Here's how the part is built. I have some questions about the finished solid (model axes, mm). Face numbers are marked on the shaded views. A direction names the side the tool comes from. Give positions to 0.01 mm unless a question says otherwise; leave off trailing zeros. Loops run counter-clockwise (first coordinate to the right, second up) from the corner with the lowest first, then second, coordinate; pieces in that order, holes last. Notation, with made-up numbers: (18.25, 55) - (30.25, 55) arc R25 cw to (30.25, 72) - close; hole circle Ø3 at (-26.75, 50). An arc over 180 degrees is marked (long way). Return JSON: item names as keys, results as strings. Group by question number.
(1) If we section it at D-D (y = 17): Please give me the cut outline in (x, z).
(2) If we section it at B-B (y = 35): Please give me the cut outline in (x, z), then the cut area to 3 significant figures.
(3) I need wall thicknesses on probe 1 along X at (y, z) = (21.5, 7.5); probe 2 along Y at (x, z) = (8, 59); probe 3 along Y at (x, z) = (32.5, 44). Which ranges of each line are inside material? Lowest first, please. Write a range as [from, to].
(4) For P1, Ø12, axis at x = 24, y = 45, coming from the +Z side; P2, Ø5, axis at x = 27, y = 8.5, coming from the +Z side; P3, Ø9.5, axis at x = 29, y = 33.5, coming from the -Z side, each with a flat end and sliding along its axis, tell me the tip position at first contact or that it passes through.
(5) If we mould it in two halves opening along Z, with no side actions, what happens to the marked faces 1, 2 and 3? For each: released by +Z, released by -Z, zero draft, split by the parting line, or undercut.
(6) If we section it at A-A (x = 30): Please give me the cut outline in (y, z), then the cut area to 3 significant figures.
(7) On a 3-axis mill with a long thin cutter (end or side, diameter ignored), from which of +Z, -Z, +X, -X, +Y, -Y can I reach the whole of each face in a straight line? I mean the marked faces 4, 5 and 6. Say none if no direction works.
(8) If we section it at C-C (z = 21.5): Please give me the cut outline in (x, y), then the cut area to 3 significant figures.
```python
from build123d import *

# Parameters (mm, degrees)
SKIZZE1_W                          = 60
SKIZZE1_H                          = 70
GRUNDK_RPER_DEPTH                  = 60
FASE2_SIZE                         = 2
WANDUNG1_T                         = -4
SKIZZE2_W                          = 20
SKIZZE2_H                          = 6
AUFSATZ_LINEAR_AUSTRAGEN1_DEPTH    = 10
BOHRUNGEN_SERVO_REACH              = 106.929
SKIZZE3_R                          = 2.5
SECHSKANT_START                    = -4.2
SKIZZE5_R                          = 2.5
SKIZZE5_R_2                        = 2
SECHSKANT_DEPTH                    = 4.2
AUSPARUNGEN_DEPTH                  = 5
FASE3_SIZE                         = 7
BOHRUNGENHALTERUNG_REACH           = 112
SKIZZE8_R                          = 2
SECHSKANT_START_2                  = -9.5
SECHSKANT_DECKEL_DEPTH             = 9.5
BOHRUNG_VERSCHRAUBUNG_DECKEL_REACH = 112
SKIZZE11_R                         = 3
SKIZZE14_W                         = 12
SKIZZE14_H                         = 20
SKIZZE14_R                         = 0.883929471
VERTIEFUNG_DECKEL_DEPTH            = 2


with BuildPart() as part:
    # Skizze1 → Grundkörper (new body)
    with BuildSketch(Plane.XY):
        with Locations((30, 35)):
            Rectangle(SKIZZE1_W, SKIZZE1_H)
    extrude(amount=GRUNDK_RPER_DEPTH)

    # Fase2
    fase2_edges = [part.edges().sort_by_distance(p)[0] for p in [
        (30, 70, 0),
        (60, 35, 0),
        (0, 35, 0),
        (0, 70, 30),
        (60, 70, 30),
        (60, 0, 30),
        (0, 0, 30),
    ]]
    chamfer(fase2_edges, length=FASE2_SIZE)

    # Wandung1
    wandung1_openings = [part.faces().sort_by_distance(p)[0] for p in [
        (30, 35, 60),
    ]]
    offset(amount=WANDUNG1_T, openings=wandung1_openings)

    # Skizze2 → Aufsatz-Linear austragen1 (add)
    with BuildSketch(Plane(origin=(0, 4, 0), x_dir=(1, 0, 0), z_dir=(0, 1, 0))):
        with Locations((30, -47.1)):
            Rectangle(SKIZZE2_W, SKIZZE2_H)
    aufsatz_linear_austragen1 = extrude(amount=AUFSATZ_LINEAR_AUSTRAGEN1_DEPTH)

    # Spiegeln1: Aufsatz-Linear austragen1 across plane
    add(aufsatz_linear_austragen1.mirror(Plane(origin=(0, 35, 0), x_dir=(0, 0, 1), z_dir=(0, -1, 0))))

    # Skizze3 → Bohrungen Servo (cut, up to next)
    with BuildSketch(Plane.XY.offset(50.1), mode=Mode.PRIVATE) as bohrungen_servo_sk1:
        with Locations((25, 9)):
            Circle(SKIZZE3_R)
    bohrungen_servo_tool1 = extrude(bohrungen_servo_sk1.sketch, amount=-BOHRUNGEN_SERVO_REACH, mode=Mode.PRIVATE) & part.part
    # Skizze3 → Bohrungen Servo (cut, up to next)
    with BuildSketch(Plane.XY.offset(50.1), mode=Mode.PRIVATE) as bohrungen_servo_sk2:
        with Locations((35, 9)):
            Circle(SKIZZE3_R)
    bohrungen_servo_tool2 = extrude(bohrungen_servo_sk2.sketch, amount=-BOHRUNGEN_SERVO_REACH, mode=Mode.PRIVATE) & part.part
    # Skizze3 → Bohrungen Servo (cut, up to next)
    with BuildSketch(Plane.XY.offset(50.1), mode=Mode.PRIVATE) as bohrungen_servo_sk3:
        with Locations((35, 61)):
            Circle(SKIZZE3_R)
    bohrungen_servo_tool3 = extrude(bohrungen_servo_sk3.sketch, amount=-BOHRUNGEN_SERVO_REACH, mode=Mode.PRIVATE) & part.part
    # Skizze3 → Bohrungen Servo (cut, up to next)
    with BuildSketch(Plane.XY.offset(50.1), mode=Mode.PRIVATE) as bohrungen_servo_sk4:
        with Locations((25, 61)):
            Circle(SKIZZE3_R)
    bohrungen_servo_tool4 = extrude(bohrungen_servo_sk4.sketch, amount=-BOHRUNGEN_SERVO_REACH, mode=Mode.PRIVATE) & part.part
    add(bohrungen_servo_tool1.solids().sort_by_distance((25, 9, 50.1))[0], mode=Mode.SUBTRACT)
    add(bohrungen_servo_tool2.solids().sort_by_distance((35, 9, 50.1))[0], mode=Mode.SUBTRACT)
    add(bohrungen_servo_tool3.solids().sort_by_distance((35, 61, 50.1))[0], mode=Mode.SUBTRACT)
    add(bohrungen_servo_tool4.solids().sort_by_distance((25, 61, 50.1))[0], mode=Mode.SUBTRACT)

    # Skizze5 → Sechskant (cut)
    # profile 1 of 4: a face of its own
    with BuildSketch(Plane(origin=(0, 0, 44.1), x_dir=(-1, 0, 0), z_dir=(0, 0, -1)).offset(SECHSKANT_START)):
        Polygon((-34.978654144, 13.041395512), (-38.489278252, 11.03918381), (-38.510624109, 6.997788298), (-35.021345856, 4.958604488), (-31.510721748, 6.96081619), (-31.489375891, 11.002211702), align=None)
        with Locations(Location((-35, 9, 0), (0, 0, 180))):
            Circle(SKIZZE5_R, mode=Mode.SUBTRACT)
    # profile 2 of 4: a face of its own
    with BuildSketch(Plane(origin=(0, 0, 44.1), x_dir=(-1, 0, 0), z_dir=(0, 0, -1)).offset(SECHSKANT_START)):
        Polygon((-31.489375891, 58.997788298), (-34.978654144, 56.958604488), (-38.489278252, 58.96081619), (-38.510624109, 63.002211702), (-35.021345856, 65.041395512), (-31.510721748, 63.03918381), align=None)
        with Locations((-35, 61)):
            Circle(SKIZZE5_R, mode=Mode.SUBTRACT)
    # profile 3 of 4: a face of its own
    with BuildSketch(Plane(origin=(0, 0, 44.1), x_dir=(-1, 0, 0), z_dir=(0, 0, -1)).offset(SECHSKANT_START)):
        Polygon((-28.489278252, 63.03918381), (-28.510624109, 58.997788298), (-25.021345856, 56.958604488), (-21.510721748, 58.96081619), (-21.489375891, 63.002211702), (-24.978654144, 65.041395512), align=None)
        with Locations((-25, 61)):
            Circle(SKIZZE5_R, mode=Mode.SUBTRACT)
    # profile 4 of 4: a face of its own
    with BuildSketch(Plane(origin=(0, 0, 44.1), x_dir=(-1, 0, 0), z_dir=(0, 0, -1)).offset(SECHSKANT_START)):
        Polygon((-28.510624109, 11.002211702), (-25.021345856, 13.041395512), (-21.510721748, 11.03918381), (-21.489375891, 6.997788298), (-24.978654144, 4.958604488), (-28.489278252, 6.96081619), align=None)
        with Locations((-25, 9)):
            Circle(SKIZZE5_R_2, mode=Mode.SUBTRACT)
    extrude(amount=SECHSKANT_DEPTH, mode=Mode.SUBTRACT)

    # Skizze7 → Ausparungen (add)
    with BuildSketch(Plane.XY.offset(60)):
        Polygon((56, 4), (41, 4), (56, 19), align=None)
        Polygon((19, 4), (4, 19), (4, 4), align=None)
        Polygon((4, 66), (19, 66), (4, 51), align=None)
        Polygon((41, 66), (56, 51), (56, 66), align=None)
    extrude(amount=-AUSPARUNGEN_DEPTH)

    # Fase3
    fase3_edges = [part.edges().sort_by_distance(p)[0] for p in [
        (56, 11.5, 55),
        (48.5, 4, 55),
        (11.5, 4, 55),
        (4, 11.5, 55),
        (4, 58.5, 55),
        (11.5, 66, 55),
        (48.5, 66, 55),
        (56, 58.5, 55),
    ]]
    chamfer(fase3_edges, length=FASE3_SIZE)

    # Skizze8 → BohrungenHalterung (cut, up to next)
    with BuildSketch(Plane.XY.offset(60), mode=Mode.PRIVATE) as bohrungenhalterung_sk1:
        with Locations((52, 8)):
            Circle(SKIZZE8_R)
    bohrungenhalterung_tool1 = extrude(bohrungenhalterung_sk1.sketch, amount=-BOHRUNGENHALTERUNG_REACH, mode=Mode.PRIVATE) & part.part
    # Skizze8 → BohrungenHalterung (cut, up to next)
    with BuildSketch(Plane.XY.offset(60), mode=Mode.PRIVATE) as bohrungenhalterung_sk2:
        with Locations(Location((8, 8, 0), (0, 0, 45))):
            Circle(SKIZZE8_R)
    bohrungenhalterung_tool2 = extrude(bohrungenhalterung_sk2.sketch, amount=-BOHRUNGENHALTERUNG_REACH, mode=Mode.PRIVATE) & part.part
    # Skizze8 → BohrungenHalterung (cut, up to next)
    with BuildSketch(Plane.XY.offset(60), mode=Mode.PRIVATE) as bohrungenhalterung_sk3:
        with Locations((8, 62)):
            Circle(SKIZZE8_R)
    bohrungenhalterung_tool3 = extrude(bohrungenhalterung_sk3.sketch, amount=-BOHRUNGENHALTERUNG_REACH, mode=Mode.PRIVATE) & part.part
    # Skizze8 → BohrungenHalterung (cut, up to next)
    with BuildSketch(Plane.XY.offset(60), mode=Mode.PRIVATE) as bohrungenhalterung_sk4:
        with Locations(Location((52, 62, 0), (0, 0, 45))):
            Circle(SKIZZE8_R)
    bohrungenhalterung_tool4 = extrude(bohrungenhalterung_sk4.sketch, amount=-BOHRUNGENHALTERUNG_REACH, mode=Mode.PRIVATE) & part.part
    add(bohrungenhalterung_tool1.solids().sort_by_distance((52, 8, 60))[0], mode=Mode.SUBTRACT)
    add(bohrungenhalterung_tool2.solids().sort_by_distance((8, 8, 60))[0], mode=Mode.SUBTRACT)
    add(bohrungenhalterung_tool3.solids().sort_by_distance((8, 62, 60))[0], mode=Mode.SUBTRACT)
    add(bohrungenhalterung_tool4.solids().sort_by_distance((52, 62, 60))[0], mode=Mode.SUBTRACT)

    # Skizze13 → Sechskant Deckel (cut)
    with BuildSketch(Plane.XY.offset(57.5).offset(SECHSKANT_START_2)):
        Polygon((50.909166509, 57.928953988), (54.98021252, 59.01978748), (56.071046012, 63.090833491), (53.090833491, 66.071046012), (49.01978748, 64.98021252), (47.928953988, 60.909166509), align=None)
        Polygon((49.01978748, 5.01978748), (53.090833491, 3.928953988), (56.071046012, 6.909166509), (54.98021252, 10.98021252), (50.909166509, 12.071046012), (47.928953988, 9.090833491), align=None)
        Polygon((3.928953988, 6.909166509), (6.909166509, 3.928953988), (10.98021252, 5.01978748), (12.071046012, 9.090833491), (9.090833491, 12.071046012), (5.01978748, 10.98021252), align=None)
        Polygon((5.01978748, 59.01978748), (9.090833491, 57.928953988), (12.071046012, 60.909166509), (10.98021252, 64.98021252), (6.909166509, 66.071046012), (3.928953988, 63.090833491), align=None)
    extrude(amount=SECHSKANT_DECKEL_DEPTH, mode=Mode.SUBTRACT)

    # Skizze11 → Bohrung Verschraubung Deckel (cut, up to next)
    with BuildSketch(Plane(origin=(0, 0, 0), x_dir=(-1, 0, 0), z_dir=(0, 0, -1)), mode=Mode.PRIVATE) as bohrung_verschraubung_deckel_sk1:
        with Locations((-30, 35)):
            Circle(SKIZZE11_R)
    bohrung_verschraubung_deckel_tool1 = extrude(bohrung_verschraubung_deckel_sk1.sketch, amount=-BOHRUNG_VERSCHRAUBUNG_DECKEL_REACH, mode=Mode.PRIVATE) & part.part
    add(bohrung_verschraubung_deckel_tool1.solids().sort_by_distance((30, 35, 0))[0], mode=Mode.SUBTRACT)

    # Skizze14 → Vertiefung Deckel (cut)
    with BuildSketch(Plane(origin=(0, 0, 0), x_dir=(-1, 0, 0), z_dir=(0, 0, -1))):
        with Locations((-30, 30)):
            Rectangle(SKIZZE14_W, SKIZZE14_H)
        with Locations((-30, 35)):
            Circle(SKIZZE14_R, mode=Mode.SUBTRACT)
    extrude(amount=-VERTIEFUNG_DECKEL_DEPTH, mode=Mode.SUBTRACT)


solid = part.part
```
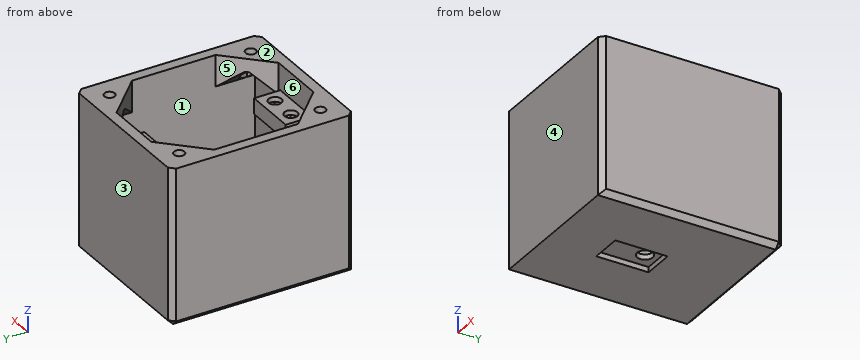
Values:
{
 "1": {"outline": "(0, 2) - (2, 0) - (58, 0) - (60, 2) - (60, 60) - (54, 60) - (54, 50) - (56, 48) - (56, 4) - (4, 4) - (4, 48) - (6, 50) - (6, 60) - (0, 60) - close"},
 "2": {"outline": "(0, 2) - (2, 0) - (24, 0) - (24, 2) - (27, 2) - (27, 4) - (4, 4) - (4, 60) - (0, 60) - close; (33, 2) - (36, 2) - (36, 0) - (58, 0) - (60, 2) - (60, 60) - (56, 60) - (56, 4) - (33, 4) - close", "area": "648 mm2"},
 "3": {"probe 1": "[0, 4], [56, 60]", "probe 2": "[0, 6], [10, 15], [55, 60], [64, 70]", "probe 3": "[0, 4], [66, 70]"},
 "4": {"P1": "z = 4", "P2": "z = 50.1", "P3": "z = 2"},
 "5": {"face 1": "undercut", "face 2": "released by +Z", "face 3": "zero draft"},
 "6": {"outline": "(0, 0) - (20, 0) - (20, 2) - (32, 2) - (32, 4) - (4, 4) - (4, 44.1) - (14, 44.1) - (14, 50.1) - (4, 50.1) - (4, 60) - (0, 60) - close; (38, 2) - (40, 2) - (40, 0) - (68, 0) - (70, 2) - (70, 60) - (66, 60) - (66, 50.1) - (56, 50.1) - (56, 44.1) - (66, 44.1) - (66, 4) - (38, 4) - close", "area": "794 mm2"},
 "7": {"face 4": "+Z, -Z, +X, -X, -Y", "face 5": "+Z", "face 6": "none"},
 "8": {"outline": "(0, 2) - (2, 0) - (58, 0) - (60, 2) - (60, 68) - (58, 70) - (2, 70) - (0, 68) - close; hole (4, 4) - (56, 4) - (56, 66) - (4, 66) - close", "area": "968 mm2"}
}
